```python
from build123d import *

# Parameters (mm, degrees)
SALIENTE_EXTRUIR1_DEPTH    = 124
SALIENTE_EXTRUIR3_START    = 5
CROQUIS7_W                 = 4
CROQUIS7_H                 = 1.5
CROQUIS7_W_2               = 2
CROQUIS7_W_3               = 1
SALIENTE_EXTRUIR3_DEPTH    = 5
CROQUIS8_W                 = 2
CROQUIS8_H                 = 1.5
CROQUIS8_W_2               = 4
SALIENTE_EXTRUIR4_DEPTH    = 5
CORTAR_EXTRUIR1_DEPTH      = 130.236217834
CORTAR_EXTRUIR1_DEPTH_BACK = 130.236217834
CROQUIS9_R                 = 1


with BuildPart() as part:
    # Croquis1 → Saliente-Extruir1 (new body)
    with BuildSketch(Plane(origin=(0, 0, 0), x_dir=(1, 0, 0), z_dir=(0, 1, 0))):
        with BuildLine():
            Line((-2, 1.5), (0, 1.5))
            Line((0, 1.5), (2, 1.5))
            ThreePointArc((2, 1.5), (3.5, 0), (2, -1.5))
            Line((2, -1.5), (1, -1.5))
            Line((1, -1.5), (1, -3))
            Line((1, -3), (2, -3))
            ThreePointArc((2, -3), (4.121320344, -2.121320344), (5, 0))
            ThreePointArc((5, 0), (4.121320344, 2.121320344), (2, 3))
            Line((2, 3), (0, 3))
            Line((0, 3), (-2, 3))
            ThreePointArc((-2, 3), (-4.121320347, 2.12132034), (-5, -9e-09))
            ThreePointArc((-5, -9e-09), (-4.12132034, -2.121320347), (-2, -3))
            Line((-2, -3), (-1, -3))
            Line((-1, -3), (-1, -1.5))
            Line((-1, -1.5), (-2, -1.5))
            ThreePointArc((-2, -1.5), (-3.5, 0), (-2, 1.5))
        make_face()
    extrude(amount=-SALIENTE_EXTRUIR1_DEPTH)

    # Croquis7 → Saliente-Extruir3 (add)
    with BuildSketch(Plane(origin=(0, 0, 0), x_dir=(1, 0, 0), z_dir=(0, 1, 0)).offset(SALIENTE_EXTRUIR3_START)):
        with Locations((0, 2.25)):
            Rectangle(CROQUIS7_W, CROQUIS7_H)
        with BuildLine():
            Line((-2, 1.5), (-2, 3))
            ThreePointArc((-2, 3), (-5, 0), (-2, -3))
            Line((-2, -3), (-2, -1.5))
            ThreePointArc((-2, -1.5), (-3.5, 0), (-2, 1.5))
        make_face()
        with Locations((0, -2.25)):
            Rectangle(CROQUIS7_W_2, CROQUIS7_H)
        with Locations((-1.5, -2.25)):
            Rectangle(CROQUIS7_W_3, CROQUIS7_H)
        with BuildLine():
            Line((2, 3), (2, 1.5))
            ThreePointArc((2, 1.5), (3.5, 0), (2, -1.5))
            Line((2, -1.5), (1, -1.5))
            Line((1, -1.5), (1, -3))
            Line((1, -3), (2, -3))
            ThreePointArc((2, -3), (5, 0), (2, 3))
        make_face()
    extrude(amount=-SALIENTE_EXTRUIR3_DEPTH)

    # Croquis8 → Saliente-Extruir4 (add)
    with BuildSketch(Plane.XZ.offset(124)):
        with BuildLine():
            Line((-2, -3), (-2, -1.5))
            ThreePointArc((-2, -1.5), (-3.5, 0), (-2, 1.5))
            Line((-2, 1.5), (-1, 1.5))
            Line((-1, 1.5), (-1, 3))
            Line((-1, 3), (-2, 3))
            ThreePointArc((-2, 3), (-5, 0), (-2, -3))
        make_face()
        with Locations((0, 2.25)):
            Rectangle(CROQUIS8_W, CROQUIS8_H)
        with BuildLine():
            Line((2, -1.5), (2, -3))
            ThreePointArc((2, -3), (5, 0), (2, 3))
            Line((2, 3), (1, 3))
            Line((1, 3), (1, 1.5))
            Line((1, 1.5), (2, 1.5))
            ThreePointArc((2, 1.5), (3.5, 0), (2, -1.5))
        make_face()
        with Locations((0, -2.25)):
            Rectangle(CROQUIS8_W_2, CROQUIS8_H)
    extrude(amount=SALIENTE_EXTRUIR4_DEPTH)

    # Croquis9 → Cortar-Extruir1 (cut, two sides: drawn at the far end of the back side and taken through both)
    with BuildSketch(Plane.XY.offset(3).offset(-CORTAR_EXTRUIR1_DEPTH_BACK)):
        with Locations((0, -126)):
            Circle(CROQUIS9_R)
    extrude(amount=CORTAR_EXTRUIR1_DEPTH + CORTAR_EXTRUIR1_DEPTH_BACK, mode=Mode.SUBTRACT)


solid = part.part
```
Geometry: final body of the model. Coordinates: model frame, mm. A direction names the side the tool comes from. Round coordinates to 2 decimals unless told otherwise and drop trailing zeros. Order: outer loops, then holes, each group sorted by start corner. A loop starts at its lowest first (then second) coordinate and runs counter-clockwise, first axis right, second up. Notation, with made-up numbers: (11, 83.25) -> (50, 83.25) arc R21 ccw to (50, 112.25) -> close; hole circle Ø8 at (85, 74). An arc over 180 degrees is marked (long way). Use one line per item in the form item = value. Start each with the question number.
1. Draft query along X for faces 1 (the face through (5, -61, 0)), 2 (the face through (-3.5, -61.1, 0)), 3 (the face through (-1.4, -61.1, 1.5)), 4 (the face through (1.4, -61.1, 3)). Return one class per face: pulls with the +X half, pulls with the -X half, needs draft (parallel to the pull), parting line crosses it, or undercut.
2. Line query: probe 1 along Y at (x, z) = (0, 2.5); probe 2 along X at (y, z) = (-39, 0.15); probe 3 along Y at (x, z) = (0, -2). Output: solid intervals per line, ascending.
3. Pin query (flat end, axial travel): pin 1 Ø1.6 at (y, z) = (-55, 2) entering from -X; pin 2 Ø2.5 at (x, y) = (0, -126) entering from -Z; pin 3 Ø0.8 at (y, z) = (-46.5, 2.5) entering from +X; pin 4 Ø2 at (y, z) = (-113.5, -1.5) entering from +X. Return the tip coordinate at first contact, or that it passes through.
4. Reachability of faces 5 (the face through (0, 5, 2)), 6 (the face through (3.5, -61.1, 0)) from +Z, -Z, +X, -X, +Y, -Y: full face, straight path, thin tool, end or side. Return the list, or none.
5. Cut plane A-A (y = -32). Return the cut outline in (x, z).
Solution:
q1.face_1 = pulls with the +X half
q1.face_2 = undercut
q1.face_3 = undercut
q1.face_4 = needs draft
q2.probe_1 = -129 to -127, -125 to -124, 0 to 5
q2.probe_2 = -5 to -3.49, 3.49 to 5
q2.probe_3 = -129 to -127, -125 to 5
q3.pin_1 = -4.75
q3.pin_2 = -3
q3.pin_3 = 4.14
q3.pin_4 = 4.96
q4.face_5 = +Z, -Z, +X, -X, +Y
q4.face_6 = +Y, -Y
q5.outline = (-2, -3) -> (2, -3) arc R3 ccw to (2, 3) -> (1, 3) -> (1, 1.5) -> (2, 1.5) arc R1.5 cw to (2, -1.5) -> (-2, -1.5) arc R1.5 cw to (-2, 1.5) -> (-1, 1.5) -> (-1, 3) -> (-2, 3) arc R3 ccw to start
